The listing builds one solid part. Answer for the finished solid, in the listing's coordinates (mm). Give positions to 0.01 mm unless a question says otherwise; leave off trailing zeros. Write each loop counter-clockwise with the first axis right and the second up, starting at its lowest first coordinate (ties: lowest second). Pieces come first, ordered by that corner, then holes. Notation, with made-up numbers: M 63,37 L 119,37 A9 ccw 119,53 Z; hole C -31,19 d7. An arc over 180 degrees is marked long. Answer as a JSON object with one key per item and string values.
```python
from build123d import *

# Parameters (mm, degrees)
F0_W     = 59.5
F0_H     = 59.5
F1_DEPTH = 2
F2_R     = 1.3
F3_R     = 5.1
F4_DEPTH = 25
F5_SIZE  = 0.4


with BuildPart() as f1:
    # F0 (on Top) → F1 (new body)
    with BuildSketch(Plane.XY):
        Rectangle(F0_W, F0_H)
    extrude(amount=F1_DEPTH)

    # F2
    f2_edges = [f1.edges().sort_by_distance(p)[0] for p in [
        (29.75, -29.75, 1),
        (-29.75, -29.75, 1),
        (29.75, 29.75, 1),
        (-29.75, 29.75, 1),
    ]]
    fillet(f2_edges, radius=F2_R)

    # F3 (on face) → F4 (cut)
    with BuildSketch(Plane.XY.offset(2)):
        Circle(F3_R)
    extrude(amount=-F4_DEPTH, mode=Mode.SUBTRACT)

    # F5
    f5_edges = [f1.edges().sort_by_distance(p)[0] for p in [
        (0, -29.75, 0),
        (-5.1, 0, 2),
        (-29.369239, -29.369239, 0),
        (29.369239, -29.369239, 0),
        (-29.75, 0, 0),
        (29.75, 0, 0),
        (-29.369239, 29.369239, 0),
        (29.369239, 29.369239, 0),
        (0, 29.75, 0),
        (-5.1, 0, 0),
    ]]
    chamfer(f5_edges, length=F5_SIZE)


solid = f1.part
```
1. A cutting plane is placed at B-B, the plane z = 1.25. Give the vertices of the cut face in (x, y), plus the area to 3 significant figures.
Verdict:
{"outline": "M -29.75,-28.45 A1.3 ccw -28.45,-29.75 L 28.45,-29.75 A1.3 ccw 29.75,-28.45 L 29.75,28.45 A1.3 ccw 28.45,29.75 L -28.45,29.75 A1.3 ccw -29.75,28.45 Z; hole C 0,0 d10.2", "area": "3,460 mm2"}
2. A cutting plane is placed at A-A, the plane x = 0. Give the vertices of the cut face in (y, z), plus the area to 3 significant figures.
Verdict:
{"outline": "M -29.75,0.4 L -29.35,0 L -5.5,0 L -5.1,0.4 L -5.1,1.6 L -5.5,2 L -29.75,2 Z; M 5.1,0.4 L 5.5,0 L 29.35,0 L 29.75,0.4 L 29.75,2 L 5.5,2 L 5.1,1.6 Z", "area": "98.1 mm2"}
3. The mould has two halves that part along X. Classify faces 1 (the cylindrical face through (29.36, -29.38, 1.21)), 2 (the cylindrical face through (2.4, -4.5, 1)), 3 (the flat face through (-29.75, 0, 1)): released by +X, released by -X, zero draft, split by the parting line, or undercut.
Verdict:
{"face 1": "released by +X", "face 2": "undercut", "face 3": "released by -X"}
4. Consider line 1 along Y through (x, z) = (0, 0.8); line 2 along Y through (x, z) = (4, 1.3); line 3 along X through (y, z) = (1, 0.55). Determine where each line is inside the solid, lowest interval first.
Verdict:
{"line 1": "y = -29.75 to -5.1, 5.1 to 29.75", "line 2": "y = -29.75 to -3.16, 3.16 to 29.75", "line 3": "x = -29.75 to -5, 5 to 29.75"}
